Design review of the part built by this model. Coordinates are the model's own, in mm. Coordinates: 2 decimals unless noted, no trailing zeros. Write each loop counter-clockwise with the first axis right and the second up, starting at its lowest first coordinate (ties: lowest second). Pieces come first, ordered by that corner, then holes. Notation, with made-up numbers: (33, -31) -> (53, -31) arc R22 cw to (53, -8) -> close; hole circle Ø8 at (-5.5, 45.5). An arc over 180 degrees is marked (long way). Answer in a Markdown table with one row per item. Add a question column.
Item 1: Take a section at D-D, the plane x = 10. Write out the cut boundary in (y, z), and give its area (3 significant figures).
Item 2: Take a section at C-C, the plane x = 82.5. Write out the cut boundary in (y, z).
Item 3: Take a section at B-B, the plane y = 1.5. Write out the cut boundary in (x, z).
Item 4: To check wall thickness, follow line 1 (X direction, y = 4.25, z = 0.25); line 2 (Y direction, x = 88.5, z = 0.25); line 3 (Y direction, x = 85, z = -1). State the ranges of each line that lie inside material, in increasing order.
Item 5: Take a section at A-A, the plane z = 0. Write out the cut boundary in (x, y).
Item 6: Clearance check with flat-ended pins moving along their axes: P1, Ø2, axis at x = 24, z = -3, coming from the +Y side; P2, Ø1, axis at x = 46, y = 4.5, coming from the -Z side; P3, Ø1.3, axis at x = 12.5, y = 5, coming from the +Z side. State where each tip first meets the part, or that it passes through.
from build123d import *

# Parameters (mm, degrees)
CUT_EXTRUDE_1_DEPTH = 2


with BuildPart() as part:
    # ｽｹｯﾁ2 → 回転1 (revolve)
    with BuildSketch(Plane.XY, mode=Mode.PRIVATE) as revolve_1_sk:
        Polygon((0, 6), (0, 0), (96.2, 0), (96.2, 6), (95.2, 6), (95.2, 5.5), (94.2, 5.5), (94.2, 6), (2, 6), (1, 6), align=None)
    revolve(revolve_1_sk.sketch.rotate(Axis((0, 0, 0), (1, 0, 0)), 90), axis=Axis((0, 0, 0), (1, 0, 0)))

    # ｽｹｯﾁ4 → ｶｯﾄ - 押し出し1 (cut)
    with BuildSketch(Plane(origin=(0, 6, 0), x_dir=(1, 0, 0), z_dir=(0, 1, 0))):
        with BuildLine():
            Line((5, 2), (15, 2))
            ThreePointArc((15, 2), (17, 0), (15, -2))
            Line((15, -2), (5, -2))
            ThreePointArc((5, -2), (3, 0), (5, 2))
        make_face()
    extrude(amount=-CUT_EXTRUDE_1_DEPTH, mode=Mode.SUBTRACT)


solid = part.part
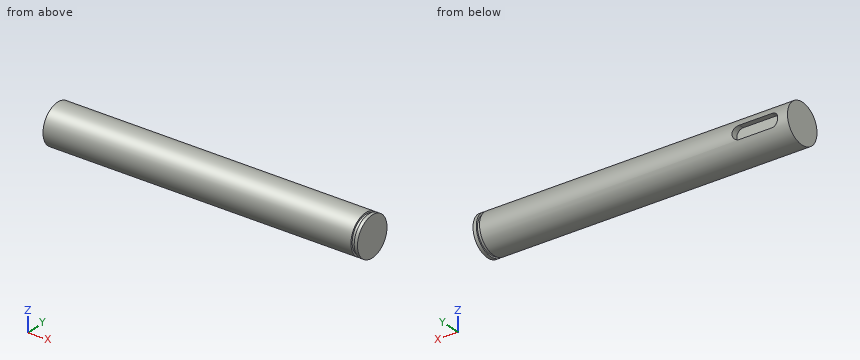
Answers:
| question | item | result |
|---|---|---|
| 1 | outline | (4, -2) -> (4, 2) -> (5.66, 2) arc R6 ccw (long way) to (5.66, -2) -> close |
| 1 | area | 106 mm^2 |
| 2 | outline | circle Ø12 at (0, 0) |
| 3 | outline | (0, -5.81) -> (94.2, -5.81) -> (94.2, -5.29) -> (95.2, -5.29) -> (95.2, -5.81) -> (96.2, -5.81) -> (96.2, 5.81) -> (95.2, 5.81) -> (95.2, 5.29) -> (94.2, 5.29) -> (94.2, 5.81) -> (0, 5.81) -> close |
| 4 | line 1 | x = 0 to 3.02, 16.98 to 96.2 |
| 4 | line 2 | y = -5.99 to 5.99 |
| 4 | line 3 | y = -5.92 to 5.92 |
| 5 | outline | (0, -6) -> (94.2, -6) -> (94.2, -5.5) -> (95.2, -5.5) -> (95.2, -6) -> (96.2, -6) -> (96.2, 6) -> (95.2, 6) -> (95.2, 5.5) -> (94.2, 5.5) -> (94.2, 6) -> (17, 6) -> (17, 4) -> (3, 4) -> (3, 6) -> (0, 6) -> close |
| 6 | P1 | stops at y = 5.66 |
| 6 | P2 | stops at z = -4.47 |
| 6 | P3 | stops at z = 4.13 |
